```python
from build123d import *

# Parameters (mm, degrees)
F1_DEPTH = 0.5
F3_DEPTH = 0.501
F5_DEPTH = 0.501


with BuildPart() as f1:
    # F0 (on Top) → F1 (new body)
    with BuildSketch(Plane.XY):
        Polygon((6.25, -10.825318), (12.5, 0), (6.25, 10.825318), (-6.25, 10.825318), (-12.5, 0), (-6.25, -10.825318), align=None)
    extrude(amount=F1_DEPTH)

    # F2 (on face) → F3 (cut, through all)
    with BuildSketch(Plane.XY.offset(0.5)):
        with BuildLine():
            ThreePointArc((4.4, -10.825318), (4.224264, -10.401053), (3.8, -10.225318))
            Line((3.8, -10.225318), (3.3, -10.225318))
            ThreePointArc((3.3, -10.225318), (2.875736, -10.401053), (2.7, -10.825318))
            Line((2.7, -10.825318), (4.4, -10.825318))
        make_face()
        with BuildLine():
            ThreePointArc((0.85, -10.825318), (0.674264, -10.401053), (0.25, -10.225318))
            Line((0.25, -10.225318), (-0.25, -10.225318))
            ThreePointArc((-0.25, -10.225318), (-0.674264, -10.401053), (-0.85, -10.825318))
            Line((-0.85, -10.825318), (0.85, -10.825318))
        make_face()
        with BuildLine():
            ThreePointArc((-2.7, -10.825318), (-2.875736, -10.401053), (-3.3, -10.225318))
            Line((-3.3, -10.225318), (-3.8, -10.225318))
            ThreePointArc((-3.8, -10.225318), (-4.224264, -10.401053), (-4.4, -10.825318))
            Line((-4.4, -10.825318), (-2.7, -10.825318))
        make_face()
    extrude(amount=-F3_DEPTH, mode=Mode.SUBTRACT)

    # F4 (on face) → F5 (cut, through all)
    with BuildSketch(Plane.XY.offset(0.5)):
        Polygon((-6.25, 10.825318), (-12.5, 0), (12.5, 0), (6.25, 10.825318), align=None)
    extrude(amount=-F5_DEPTH, mode=Mode.SUBTRACT)


solid = f1.part
```
Could you check a few things on this model? Use its own coordinates, in mm. Coordinates: 2 decimals unless noted, no trailing zeros. Loops run counter-clockwise (first coordinate to the right, second up) from the corner with the lowest first, then second, coordinate; pieces in that order, holes last. Notation, with made-up numbers: M 17,23.5 L 44,23.5 A32 ccw 44,60.5 Z; hole C 57.25,46.5 d2. An arc over 180 degrees is marked long. Put each result on its own line as item: value. Start each with the question number.
(1) I need wall thicknesses on line 1 (Y direction, x = 0, z = 0.05); line 2 (X direction, y = -0.75, z = 0.15); line 3 (X direction, y = -10, z = 0.45). Which ranges of each line are inside material? Lowest first, please. Write a range as from..to.
(2) Thinking about a two-plate mould opening in Y: for faces 1 (the face through (0, -4, 0.5)), 2 (the face through (-9.419, -5.337, 0.246)), which applies, pulls with the +Y half, pulls with the -Y half, needs draft (parallel to the pull), parting line crosses it, or undercut?
(3) Suppose I cut it at A-A on z = 0.3. Please give me the cut outline in (x, y).
(4) Suppose I cut it at B-B on y = -1.25. Please give me the cut outline in (x, z).
(5) Suppose I cut it at C-C on x = -3. Please give me the cut outline in (y, z).
Solutions:
1. line 1: y = -10.23..0
1. line 2: x = -12.07..12.07
1. line 3: x = -6.73..6.73
2. face 1: needs draft
2. face 2: pulls with the -Y half
3. outline: M -12.5,0 L -6.25,-10.83 L -4.4,-10.83 A0.6 cw -3.8,-10.23 L -3.3,-10.23 A0.6 cw -2.7,-10.83 L -0.85,-10.83 A0.6 cw -0.25,-10.23 L 0.25,-10.23 A0.6 cw 0.85,-10.83 L 2.7,-10.83 A0.6 cw 3.3,-10.23 L 3.8,-10.23 A0.6 cw 4.4,-10.83 L 6.25,-10.83 L 12.5,0 Z
4. outline: M -11.78,0 L 11.78,0 L 11.78,0.5 L -11.78,0.5 Z
5. outline: M -10.31,0 L 0,0 L 0,0.5 L -10.31,0.5 Z
